from build123d import *

# Parameters (mm, degrees)
CUT_EXTRUDE_1_REACH = 10.372


with BuildPart() as part:
    # 草图1 → 旋转1 (revolve)
    with BuildSketch(Plane.XY, mode=Mode.PRIVATE) as revolve_1_sk:
        Polygon((2, 0), (2, 3.75), (1.75, 4), (0, 4), (0, 0), (1.25, -0.751075774), (1.25, -1.9), (3.067834087, -1.9), (4.2, -0.95), (4.2, 0), align=None)
    revolve(revolve_1_sk.sketch.rotate(Axis((0, 0, 0), (0, 1, 0)), 90), axis=Axis((0, 0, 0), (0, 1, 0)))

    # 切除-拉伸1: up to this cone (the profile starts inside it)
    cut_extrude_1_end = Plane(origin=(0, -1.9, 0), z_dir=(0, -1, 0)).offset(-1.899999) * Cone(1.664e-06, 26.51884732, 15.934130016, align=(Align.CENTER, Align.CENTER, Align.MIN), mode=Mode.PRIVATE)
    # 草图2 → 切除-拉伸1 (cut, up to the surface)
    with BuildSketch(Plane.XZ.offset(1.9), mode=Mode.PRIVATE) as cut_extrude_1_sk1:
        Polygon((1.443375673, 0), (0.721687836, 1.25), (-0.721687836, 1.25), (-1.443375673, 0), (-0.721687836, -1.25), (0.721687836, -1.25), align=None)
    cut_extrude_1_tool1 = extrude(cut_extrude_1_sk1.sketch, amount=-CUT_EXTRUDE_1_REACH, mode=Mode.PRIVATE) & cut_extrude_1_end
    add(cut_extrude_1_tool1.solids().sort_by_distance((0, -1.9, 0))[0], mode=Mode.SUBTRACT)


solid = part.part
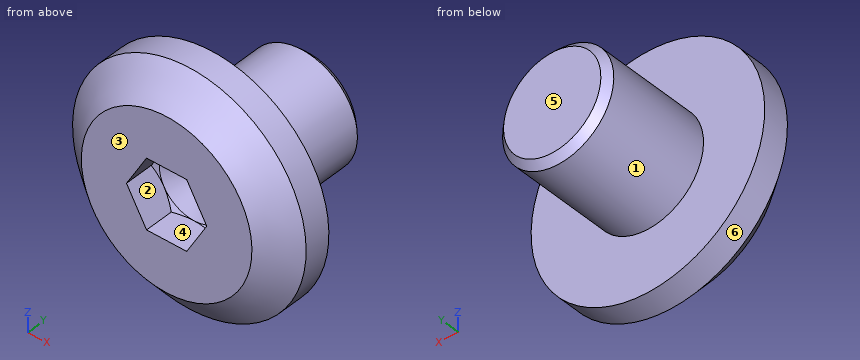
Read the model definition and answer for the solid it produces. Units are mm, in the model's axes. Face numbers are marked on the shaded views. A direction names the side the tool comes from. Round coordinates to 2 decimals unless told otherwise and drop trailing zeros. Write each loop counter-clockwise with the first axis right and the second up, starting at its lowest first coordinate (ties: lowest second). Pieces come first, ordered by that corner, then holes. Notation, with made-up numbers: (-25.75, 68.25) - (3.25, 68.25) arc R14 ccw to (3.25, 81.25) - close; hole circle Ø9 at (50, 55.5). An arc over 180 degrees is marked (long way). Use a Markdown table: item, result.
(1) The mould has two halves that part along Z. Classify the marked faces 4, 5 and 6: released by +Z, released by -Z, zero draft, split by the parting line, or undercut.
Reported:
| item | result |
|---|---|
| face 4 | undercut |
| face 5 | zero draft |
| face 6 | split by the parting line |
(2) Each of these flat-tipped pins is pushed along its axis until it touches: pin 1 Ø1 at (x, y) = (3, 2) entering from -Z; pin 2 Ø0.6 at (x, y) = (0, -1.5) entering from +Z; pin 3 Ø1.5 at (y, z) = (0, 1) entering from -X; pin 4 Ø3 at (x, y) = (2.5, -1) entering from +Z. Where does it stop, or does it pass through?
Reported:
| item | result |
|---|---|
| pin 1 | through |
| pin 2 | z = 3.9 |
| pin 3 | x = -4.19 |
| pin 4 | z = 4.08 |
(3) Straight lines are drawn through the part: line 1 along Y through (x, z) = (2.25, -0.25); line 2 along Z through (x, y) = (-0.25, -1.1); line 3 along X through (y, z) = (-0.35, -2.5). For each, find the intervals that lie inside material, in ascending order. Write a range as [from, to].
Reported:
| item | result |
|---|---|
| line 1 | [-1.9, 0] |
| line 2 | [-4.01, -1.25], [1.25, 4.01] |
| line 3 | [-3.37, 3.37] |
(4) Which of the six approach directions +Z, -Z, +X, -X, +Y, -Y give full straight-line access (tool end or side, diameter ignored) to the marked faces 1, 2 and 3?
Reported:
| item | result |
|---|---|
| face 1 | +Y |
| face 2 | -Y |
| face 3 | +Z, -Z, +X, -X, -Y |
(5) The part is cut by section B-B (y = 2). Write down the section's boundary in (x, z), then the cut area to 3 significant figures.
Reported:
| item | result |
|---|---|
| outline | circle Ø4 at (0, 0) |
| area | 12.6 mm2 |
(6) The part is cut by section A-A (y = -0.2). Write down the section's boundary in (x, z).
Reported:
| item | result |
|---|---|
| outline | circle Ø8.4 at (0, 0); hole circle Ø0.67 at (0, 0) |
